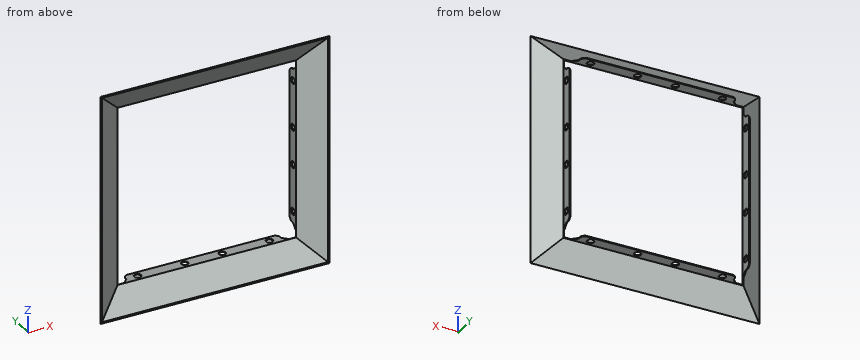
from build123d import *

# Parameters (mm, degrees)
F0_W      = 300
F0_H      = 300
F2_W      = 237
F2_H      = 237
F5_W      = 237
F5_H      = 237
F3_FACE_W = 237
F3_FACE_H = 237
F7_T      = 1
F14_R     = 4.5
F15_DEPTH = 271.3666433207
F16_R     = 4.5
F17_DEPTH = 271.3666433207


with BuildPart() as f3:
    # F0 (on Front) → F3 section 0
    with BuildSketch(Plane.XZ):
        Rectangle(F0_W, F0_H)
    # F2 (on offset) → F3 section 1
    with BuildSketch(Plane.XZ.offset(-20)):
        Rectangle(F2_W, F2_H)
    loft()

    # F5 (on offset) → F6 section 0
    with BuildSketch(Plane.XZ.offset(-36)):
        Rectangle(F5_W, F5_H)
    # F3_face (on face) → F6 section 1
    with BuildSketch(Plane(origin=(0, 20, 0), x_dir=(-1, 0, 0), z_dir=(0, 1, 0))):
        Rectangle(F3_FACE_W, F3_FACE_H)
    loft()

    # F7
    f7_openings = [f3.faces().sort_by_distance(p)[0] for p in [
        (0, 0, 0),
        (0, 36, 0),
    ]]
    offset(amount=F7_T, openings=f7_openings, kind=Kind.INTERSECTION)

    # F8 (on face) → F9 (revolve, cut)
    with BuildSketch(Plane(origin=(-119.5, 0, 0), x_dir=(0, -1, 0), z_dir=(-1, 0, 0))):
        with BuildLine():
            Line((-20.5496148068, 109.5), (-20.5496148068, 119.5))
            Line((-20.5496148068, 119.5), (-36, 119.5))
            Line((-36, 119.5), (-36, 96.9205275363))
            ThreePointArc((-36, 96.9205275363), (-33.0609608371, 101.5771569003), (-27.6206826186, 102.4289321881))
            Line((-27.6206826186, 102.4289321881), (-20.5496148068, 109.5))
        make_face()
    revolve(axis=Axis((-119.5, 28.2748074034, 119.5), (0, 1, 0)), mode=Mode.SUBTRACT)

    # F8 (on face) → F10 (revolve, cut)
    with BuildSketch(Plane(origin=(-119.5, 0, 0), x_dir=(0, -1, 0), z_dir=(-1, 0, 0))):
        with BuildLine():
            Line((-36, -119.5), (-20.5496148068, -119.5))
            Line((-20.5496148068, -119.5), (-20.5496148068, -109.5))
            Line((-20.5496148068, -109.5), (-27.6206826186, -102.4289321881))
            ThreePointArc((-27.6206826186, -102.4289321881), (-33.0609608371, -101.5771569003), (-36, -96.9205275363))
            Line((-36, -96.9205275363), (-36, -119.5))
        make_face()
    revolve(axis=Axis((-119.5, 28.2748074034, -119.5), (0, 1, 0)), mode=Mode.SUBTRACT)

    # F11 (on face) → F12 (revolve, cut)
    with BuildSketch(Plane.YZ.offset(119.5)):
        with BuildLine():
            Line((27.6206826186, -102.4289321881), (20.5496148068, -109.5))
            Line((20.5496148068, -109.5), (20.5496148068, -119.5))
            Line((20.5496148068, -119.5), (36, -119.5))
            Line((36, -119.5), (36, -96.9205275363))
            ThreePointArc((36, -96.9205275363), (33.0609608371, -101.5771569003), (27.6206826186, -102.4289321881))
        make_face()
    revolve(axis=Axis((119.5, 28.2748074034, -119.5), (0, 1, 0)), mode=Mode.SUBTRACT)

    # F11 (on face) → F13 (revolve, cut)
    with BuildSketch(Plane.YZ.offset(119.5)):
        with BuildLine():
            Line((36, 119.5), (20.5496148068, 119.5))
            Line((20.5496148068, 119.5), (20.5496148068, 109.5))
            Line((20.5496148068, 109.5), (27.6206826186, 102.4289321881))
            ThreePointArc((27.6206826186, 102.4289321881), (33.0609608371, 101.5771569003), (36, 96.9205275363))
            Line((36, 96.9205275363), (36, 119.5))
        make_face()
    revolve(axis=Axis((119.5, 28.2748074034, 119.5), (0, 1, 0)), mode=Mode.SUBTRACT)

    # F14 (on face) → F15 (cut, through all)
    with BuildSketch(Plane(origin=(0, 0, -119.5), x_dir=(1, 0, 0), z_dir=(0, 0, -1))):
        with Locations((-25, -28)):
            Circle(F14_R)
        with Locations((25, -28)):
            Circle(F14_R)
        with Locations((-87.5, -28)):
            Circle(F14_R)
        with Locations((87.5, -28)):
            Circle(F14_R)
    extrude(amount=-F15_DEPTH, mode=Mode.SUBTRACT)

    # F16 (on face) → F17 (cut, through all)
    with BuildSketch(Plane(origin=(-119.5, 0, 0), x_dir=(0, -1, 0), z_dir=(-1, 0, 0))):
        with Locations((-28, 25)):
            Circle(F16_R)
        with Locations((-28, 87.5)):
            Circle(F16_R)
        with Locations((-28, -25)):
            Circle(F16_R)
        with Locations((-28, -87.5)):
            Circle(F16_R)
    extrude(amount=-F17_DEPTH, mode=Mode.SUBTRACT)


solid = f3.part
Part model, mm, in its own coordinate system. Give positions to 0.01 mm unless a question says otherwise; leave off trailing zeros. Write each question's results on one line, items separated by ' | '. Start each with the question number.
Q1. Wall check: L1, parallel to X at y = 24, z = 59; L2, parallel to Z at x = 118.8, y = 28; L3, parallel to X at y = 28, z = -119.05. Give the ranges that are in metal, low to high.
Q2. Band-saw the part on A-A on z = 25. Count the separate pieces of the cut face and the enclosed holes in it, plus the area to 3 significant figures.
Q3. Pin check, flat tips, straight feed: P1, Ø14.5, axis at y = 28, z = 87.5, coming from the +X side; P2, Ø10.5, axis at x = -25, y = 28, coming from the +Z side; P3, Ø6, axis at y = 12.5, z = -22, coming from the -X side. Stop position of each tip, or through.
Results are:
1) L1: x = -119.5 to -118.5, 118.5 to 119.5 | L2: z = -102.54 to -92, -83 to -29.5, -20.5 to 20.5, 29.5 to 83, 92 to 102.54 | L3: x = -102.53 to -92, -83 to -29.5, -20.5 to 20.5, 29.5 to 83, 92 to 102.53
2) separate pieces: 4 | enclosed holes: 0 | area: 89.1 mm²
3) P1: stops at x = 119.5 | P2: stops at z = 119.5 | P3: stops at x = -136.9
